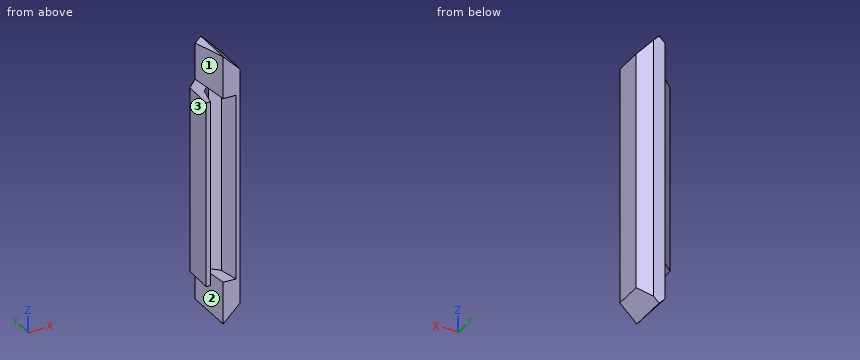
Autodesk Inventor part; units mm, degrees
ref_plane "YZ Plane" through (0, 0, 0) normal (1, 0, 0) x (0, 1, 0)
ref_plane "XZ Plane" through (0, 0, 0) normal (0, 1, 0) x (-1, 0, 0)
ref_plane "XY Plane" through (0, 0, 0) normal (0, 0, 1) x (1, 0, 0)
sketch "Sketch1" plane through (0, 0, 0) normal (0, 0, 1) x (1, 0, 0)
  line L0 (6, 0) -> (6, 11)
  line L1 (0, 15) -> (2, 15)
  line L2 (2, 15) -> (6, 11)
  line L3 (0, 10) -> (3, 7)
  line L4 (-6, 0) -> (-6, 11)
  line L5 (0, 15) -> (-2, 15)
  line L6 (-2, 15) -> (-6, 11)
  line L7 (0, 10) -> (-3, 7)
  line L8 (-4.5, 0) -> (-3, 7)
  line L9 (3, 7) -> (4.5, 0)
  line L10 (-6, 0) -> (-4.5, 0)
  line L11 (4.5, 0) -> (6, 0)
  point P0 (0, 0)
  dimension "d2" = 11
  dimension "d4" = 2
  dimension "d5" = 10
extrude "Extrusion1" add sketch "Sketch1" along normal blind 66
sketch "Sketch2" plane through (0, 0, 66) normal (0, 0, 1) x (1, 0, 0)
  line L0 (2, 15) -> (-2, 15)
  line L1 (0, 15) -> (2, 15)
  line L2 (6, 11) -> (2, 15)
  line L3 (4.5, 0) -> (6, 0)
  line L4 (0, 0) -> (6, 0)
  line L5 (6, 0) -> (6, 11)
  line L6 (6, 0) -> (6, 11)
  line L7 (6, 11) -> (2, 15)
  line L8 (0, 15) -> (-2, 15)
  line L9 (-2, 15) -> (0, 0)
extrude "Extrusion2" add sketch "Sketch2" along normal blind 15
sketch "Sketch5" plane through (0, 0, 0) normal (0, 0, -1) x (-1, 0, 0)
  line L0 (0, 0) -> (-6, 0)
  line L1 (-6, 0) -> (-6, 11)
  line L2 (-6, 11) -> (-2, 15)
  line L3 (-2, 15) -> (2, 15)
  line L4 (2, 15) -> (0, 0)
extrude "Extrusion4" add sketch "Sketch5" along normal blind 15
sketch "Sketch6" plane through (0, 0, 66) normal (0, -1, 0) x (1, 0, 0)
  line L0 (0, -66) -> (0, -81)
  line L1 (6, -81) -> (6, 15)
  line L2 (0, -81) -> (6, -81)
  line L3 (6, -81) -> (6, -75)
  line L4 (6, -75) -> (0, -81)
  line L5 (-2, -81) -> (2, -81)
  line L6 (0, -81) -> (-2, -81)
  line L7 (-2, -81) -> (-2, -79)
  line L8 (-2, -66) -> (-2, -81)
  line L9 (-2, -79) -> (0, -81)
  line L10 (2, 15) -> (-2, 15)
  line L11 (6, 15) -> (2, 15)
  line L12 (0, 15) -> (6, 15)
  line L13 (6, 15) -> (6, 9)
  line L14 (0, 0) -> (0, 15)
  line L15 (6, 9) -> (0, 15)
  line L16 (0, 15) -> (-2, 15)
  line L17 (-2, 0) -> (-2, 15)
  line L18 (-2, 15) -> (-2, 13)
  line L19 (-2, 13) -> (0, 15)
  dimension "d16" = 6
  dimension "d17" = 2
  dimension "d18" = 6
extrude "Extrusion5" cut sketch "Sketch6" against normal blind 37.3875
properties part number "outside-join-2"
CAD build for the part. Positions are in the model's coordinates, mm. Face numbers are marked on the shaded views. A direction names the side the tool comes from. Give positions to 0.01 mm unless a question says otherwise; leave off trailing zeros. Write each loop counter-clockwise with the first axis right and the second up, starting at its lowest first coordinate (ties: lowest second). Pieces come first, ordered by that corner, then holes. Notation, with made-up numbers: (62.25, 55) - (72.25, 55) arc R19 cw to (72.25, 74) - close; hole circle Ø1 at (-13, -7.5). An arc over 180 degrees is marked (long way). Put each result on its own line as item: value.
(1) Wall check: L1, parallel to Z at x = 0, y = 6; L2, parallel to X at y = 9.5, z = 14; L3, parallel to Z at x = 2, y = 4. Give the ranges that are in metal, low to high.
Working result:
L1: -15 to 0, 66 to 81
L2: -6 to -0.5, 0.5 to 6
L3: -13 to 0, 66 to 79
(2) Saw through at A-A (z = 24.5). List the corners of the cut face in (x, y), then the cut area to 4 significant figures.
Working result:
outline: (-6, 0) - (-4.5, 0) - (-3, 7) - (0, 10) - (3, 7) - (4.5, 0) - (6, 0) - (6, 11) - (2, 15) - (-2, 15) - (-6, 11) - close
area: 102.5 mm^2
(3) Saw through at C-C (y = 6). List the corners of the cut face in (x, z), then the cut area to 3 significant figures.
Working result:
outline: (-6, 0) - (-3.21, 0) - (-3.21, 66) - (-6, 66) - close; (-0.8, -14.2) - (0, -15) - (6, -9) - (6, 75) - (0, 81) - (-0.8, 80.2) - (-0.8, 66) - (3.21, 66) - (3.21, 0) - (-0.8, 0) - close
area: 535 mm^2
(4) Tool access for the marked faces 1, 2 and 3: list every direction of +Z, -Z, +X, -X, +Y, -Y with a clear straight run to the whole face (end or side of a thin tool).
Working result:
face 1: +Z, -X, -Y
face 2: -Z, -X, -Y
face 3: +Z, -Z, -X, +Y, -Y
(5) Drop flat-ended pins along their axis: pin 1 Ø4.5 at (x, y) = (1, 5.5) entering from -Z; pin 2 Ø5.5 at (x, y) = (-4.5, 5.5) entering from -Z; pin 3 Ø4 at (x, y) = (-3, 9.5) entering from +Z. Give the stop position or say it passes through.
Working result:
pin 1: z = -15
pin 2: z = 0
pin 3: z = 80
(6) Saw through at D-D (z = -2). List the corners of the cut face in (x, y), then the cut area to 3 significant figures.
Working result:
outline: (-2, 15) - (0, 0) - (6, 0) - (6, 11) - (2, 15) - close
area: 97.0 mm^2
(7) Saw through at B-B (y = 2). List the corners of the cut face in (x, z), then the cut area to 4 significant figures.
Working result:
outline: (-6, 0) - (-4.07, 0) - (-4.07, 66) - (-6, 66) - close; (-0.27, -14.73) - (0, -15) - (6, -9) - (6, 75) - (0, 81) - (-0.27, 80.73) - (-0.27, 66) - (4.07, 66) - (4.07, 0) - (-0.27, 0) - close
area: 406.5 mm^2
